Can you work these out from the model? Positions are in its coordinate system, mm. A direction names the side the tool comes from. Round coordinates to 2 decimals unless told otherwise and drop trailing zeros. Loops run counter-clockwise (first coordinate to the right, second up) from the corner with the lowest first, then second, coordinate; pieces in that order, holes last. Notation, with made-up numbers: M 52,26.25 L 93,26.25 A25 cw 93,64.25 Z; hole C 21,-30 d7. An arc over 180 degrees is marked long. Use a Markdown table: item, result. Add a question column.
```python
from build123d import *

# Parameters (mm, degrees)
SKETCH3_W           = 23
SKETCH3_H           = 12.2
BOSS_EXTRUDE1_DEPTH = 3
CUT_EXTRUDE1_DEPTH  = 79.334093387
SKETCH6_W           = 12.2
SKETCH6_H           = 3
BOSS_EXTRUDE2_DEPTH = 14.35


with BuildPart() as part:
    # Sketch3 → Boss-Extrude1 (new body)
    with BuildSketch(Plane(origin=(0, 0, 0), x_dir=(1, 0, 0), z_dir=(0, 1, 0))):
        with BuildLine():
            Line((-16.25, 9.2), (16.25, 9.2))
            ThreePointArc((16.25, 9.2), (45.532149663, 0.13158895), (76.073056463, -2.501542212))
            ThreePointArc((76.073056463, -2.501542212), (77.734099253, -4.472609946), (76.073056463, -6.443677679))
            ThreePointArc((76.073056463, -6.443677679), (46.188824578, -8.36062795), (16.25, -9))
            Line((16.25, -9), (-16.25, -9))
            Line((-16.25, -9), (-16.25, 9.2))
        make_face()
        with Locations((0.25, 0.1)):
            Rectangle(SKETCH3_W, SKETCH3_H, mode=Mode.SUBTRACT)
    extrude(amount=BOSS_EXTRUDE1_DEPTH)

    # Sketch5 → Cut-Extrude1 (cut, through all)
    with BuildSketch(Plane(origin=(0, 3, 0), x_dir=(1, 0, 0), z_dir=(0, 1, 0))):
        with BuildLine():
            Line((19.25, 4.714006378), (19.25, -4.579341889))
            Line((19.25, -4.579341889), (25.977749381, 2.242895118))
            ThreePointArc((25.977749381, 2.242895118), (22.598740451, 3.437246869), (19.25, 4.714006378))
        make_face()
        with BuildLine():
            Line((20.671769547, -5.985999467), (26.990590291, 0.332821278))
            Line((26.990590291, 0.332821278), (33.119603604, -5.796192035))
            ThreePointArc((33.119603604, -5.796192035), (26.896109589, -5.918837556), (20.671769547, -5.985999467))
        make_face()
        with BuildLine():
            Line((35.952850124, -5.721969404), (38.698754677, -2.976064852))
            Line((38.698754677, -2.976064852), (41.274144832, -5.551455007))
            ThreePointArc((41.274144832, -5.551455007), (38.613659992, -5.64178383), (35.952850124, -5.721969404))
        make_face()
        with BuildLine():
            Line((44.109524036, -5.444008267), (46.395047974, -3.086577857))
            ThreePointArc((46.395047974, -3.086577857), (52.157632807, -4.035426025), (57.95349503, -4.753533193))
            ThreePointArc((57.95349503, -4.753533193), (51.033222886, -5.133123327), (44.109524036, -5.444008267))
        make_face()
        with BuildLine():
            Line((29.11239722, 1.217185885), (34.499115549, -4.347276855))
            Line((34.499115549, -4.347276855), (37.58866149, -1.173111994))
            ThreePointArc((37.58866149, -1.173111994), (33.332539672, -0.041756487), (29.11239722, 1.217185885))
        make_face()
        with BuildLine():
            Line((40.562529295, -1.882957729), (42.638111064, -4.086994114))
            Line((42.638111064, -4.086994114), (44.022530764, -2.626821374))
            ThreePointArc((44.022530764, -2.626821374), (42.290280718, -2.265351983), (40.562529295, -1.882957729))
        make_face()
    extrude(amount=-CUT_EXTRUDE1_DEPTH, mode=Mode.SUBTRACT)

    # Sketch6 → Boss-Extrude2 (add)
    with BuildSketch(Plane.XZ):
        with Locations((-5.15, 7.5)):
            Rectangle(SKETCH6_W, SKETCH6_H)
    extrude(amount=BOSS_EXTRUDE2_DEPTH)


solid = part.part
```
(1) Suppose I cut it at A-A on x = -0.5. List the corners of the cut face in (y, z) for me, and give its area (4 significant figures).
(2) Suppose I cut it at B-B on x = 22.5. List the corners of the cut face in (y, z) for me, and give its area (3 significant figures).
(3) On a 3-axis mill with a long thin cutter (end or side, diameter ignored), from which of +Z, -Z, +X, -X, +Y, -Y can I reach the whole of each face in a straight line? I mean faces 1 (the face through (46.608, 1.479, 8.343)), 2 (the face through (36.022, 1.521, 2.782)). Say none if no direction works.
(4) I'm going to push flat-ended pins straight in: pin 1 (2.5 mm diameter, centred on y = 2, z = 2, fed in from +X); pin 2 (5.5 mm diameter, centred on x = 43, z = -2, fed in from -Y); pin 3 (0.9 mm diameter, centred on y = -9, z = 8, fed in from -X). Where does each tip first touch, or does it pass through?
(5) Suppose I cut it at C-C on z = 7.75. List the corners of the cut face in (x, y) for me, and give its area (3 significant figures).
(6) Suppose I cut it at D-D on y = -9.5. List the corners of the cut face in (x, z) for me.
(7) Thinking about a two-plate mould opening in X: for faces 3 (the face through (-5, -14.35, 8)), 4 (the face through (43.32, 1.52, 3.37)), 5 (the face through (-2, -4, 6)), 6 (the face through (-11.25, -7, 7)), which applies, released by +X, released by -X, zero draft, split by the parting line, or undercut?
(8) If I drill on probe 1 along Y at (x, z) = (27.5, -3.5); probe 2 along Z at (x, y) = (-9.5, -11.25); probe 3 along Z at (x, y) = (4, 1), over which ranges is the centre line in solid material (lowest first)? Write a range as [from, to].
Results below:
| question | item | result |
|---|---|---|
| 1 | outline | M -14.35,6 L 3,6 L 3,9 L -14.35,9 Z; M 0,-9.2 L 3,-9.2 L 3,-6.2 L 0,-6.2 Z |
| 1 | area | 61.05 mm² |
| 2 | outline | M 0,-6.67 L 3,-6.67 L 3,-3.47 L 0,-3.47 Z; M 0,1.28 L 3,1.28 L 3,4.16 L 0,4.16 Z; M 0,5.97 L 3,5.97 L 3,8.97 L 0,8.97 Z |
| 2 | area | 27.2 mm² |
| 3 | face 1 | +Z, +X, +Y, -Y |
| 3 | face 2 | +Y, -Y |
| 4 | pin 1 | stops at x = 77.32 |
| 4 | pin 2 | stops at y = 0 |
| 4 | pin 3 | stops at x = -11.25 |
| 5 | outline | M -16.25,0 L -11.25,0 L -11.25,-14.35 L 0.95,-14.35 L 0.95,0 L 58.1,0 L 58.1,3 L -16.25,3 Z |
| 5 | area | 398 mm² |
| 6 | outline | M -11.25,6 L 0.95,6 L 0.95,9 L -11.25,9 Z |
| 7 | face 3 | zero draft |
| 7 | face 4 | undercut |
| 7 | face 5 | undercut |
| 7 | face 6 | released by -X |
| 8 | probe 1 | y = [0, 3] |
| 8 | probe 2 | z = [6, 9] |
| 8 | probe 3 | z = [-9.2, -6.2], [6, 9] |
